Could you check a few things on this model? Use its own coordinates, in mm. Face numbers are marked on the shaded views. A direction names the side the tool comes from. Give positions to 0.01 mm unless a question says otherwise; leave off trailing zeros. Loops run counter-clockwise (first coordinate to the right, second up) from the corner with the lowest first, then second, coordinate; pieces in that order, holes last. Notation, with made-up numbers: (88.25, 43) -> (105.25, 43) arc R16 ccw to (105.25, 50) -> close; hole circle Ø3 at (75, 75.5). An arc over 180 degrees is marked (long way). Put each result on its own line as item: value.
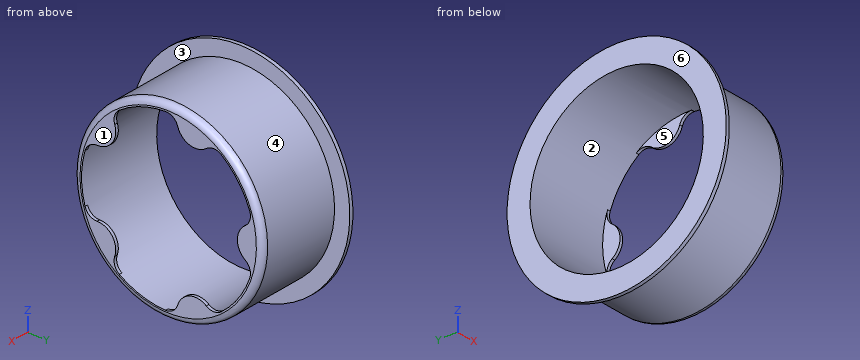
```python
from build123d import *

# Parameters (mm, degrees)
SKETCH_3_R          = 19
CUT_EXTRUDE_1_DEPTH = 0.6
EXTRUDE_1_DEPTH     = 0.5
FILLET_1_R          = 2
FILLET_2_R          = 1


with BuildPart() as part:
    # 草图2 → 旋转1 (revolve)
    with BuildSketch(Plane(origin=(0, 0, 0), x_dir=(1, 0, 0), z_dir=(0, 1, 0)), mode=Mode.PRIVATE) as revolve_1_sk:
        Polygon((-7.6, 14.15), (-7.6, 17.9), (-7, 17.9), (-7, 15.4), (7, 15.4), (7, 17.9), (7.6, 17.9), (7.6, 14.15), align=None)
    revolve(revolve_1_sk.sketch.rotate(Axis((-68.553057404, 0, 0), (1, 0, 0)), 180), axis=Axis((-68.553057404, 0, 0), (1, 0, 0)))

    # 草图3 → 切除-拉伸1 (cut)
    with BuildSketch(Plane(origin=(7.6, 0, 0), x_dir=(0, 0, -1), z_dir=(1, 0, 0))):
        Circle(SKETCH_3_R)
    extrude(amount=-CUT_EXTRUDE_1_DEPTH, mode=Mode.SUBTRACT)

    # 草图4 → 凸台-拉伸1 (add)
    with BuildSketch(Plane(origin=(7, 0, 0), x_dir=(0, 0, -1), z_dir=(1, 0, 0))):
        with BuildLine():
            ThreePointArc((-12.378887951, 7.159129353), (-13.600108183, 4.41894302), (-14.222761377, 1.484270465))
            ThreePointArc((-14.222761377, 1.484270465), (-10.746938634, 3.491892036), (-12.378887951, 7.159129353))
        make_face()
        with BuildLine():
            ThreePointArc((-2.983449874, 13.985314685), (0, 11.3), (2.983449874, 13.985314685))
            ThreePointArc((2.983449874, 13.985314685), (0, 14.3), (-2.983449874, 13.985314685))
        make_face()
        with BuildLine():
            ThreePointArc((12.378887951, 7.159129353), (10.746938634, 3.491892036), (14.222761377, 1.484270465))
            ThreePointArc((14.222761377, 1.484270465), (13.600108183, 4.41894302), (12.378887951, 7.159129353))
        make_face()
        with BuildLine():
            ThreePointArc((10.634023371, -9.560729415), (6.641973351, -9.141892036), (5.80670007, -13.067985089))
            ThreePointArc((5.80670007, -13.067985089), (8.405329108, -11.56894302), (10.634023371, -9.560729415))
        make_face()
        with BuildLine():
            ThreePointArc((-5.80670007, -13.067985089), (-6.641973351, -9.141892036), (-10.634023371, -9.560729415))
            ThreePointArc((-10.634023371, -9.560729415), (-8.405329108, -11.56894302), (-5.80670007, -13.067985089))
        make_face()
    extrude(amount=-EXTRUDE_1_DEPTH)

    # 圆角1
    # the kernel refuses this fillet: 2 mm, written as the material it adds along each edge
    with BuildSketch(Plane(origin=(7, 13.836101399, -2.963916005), x_dir=(0, -0.2740436561087124, -0.9617172529109426), z_dir=(-1, 0, 0)), Plane(origin=(7, 1.456738837, -14.074814811), x_dir=(0, -0.9993316071526622, -0.03655597004153086), z_dir=(-1, 0, 0)), Plane(origin=(7, -12.935787284, -5.734797933), x_dir=(0, -0.3435772431436893, 0.9391244209335534), z_dir=(-1, 0, 0)), Plane(origin=(7, -9.45149505, 10.53051477), x_dir=(0, 0.7869891931288754, 0.6169667818435298), z_dir=(-1, 0, 0)), Plane(origin=(7, 7.094442099, 12.24301398), x_dir=(0, 0.8299633132761892, -0.5578179798246109), z_dir=(-1, 0, 0))) as fillet_1_piece_1:
        with BuildLine():
            CenterArc((1.749454913, 1.995570291), FILLET_1_R, 199.01971257, 74.794373043)
            ThreePointArc((-0.141358103, 1.34378341), (0.005960171, 0.6799537), (0, 0))
            ThreePointArc((0, 0), (0.941246655, -0.031340193), (1.88249331, 0))
        make_face()
    extrude(amount=0.5)
    with BuildSketch(Plane(origin=(7, 13.836101399, 2.963916005), x_dir=(0, -0.2740436561087127, 0.9617172529109423), z_dir=(-1, 0, 0)), Plane(origin=(7, 7.094442099, -12.24301398), x_dir=(0, 0.8299633132761899, 0.5578179798246101), z_dir=(-1, 0, 0)), Plane(origin=(7, -9.45149505, -10.53051477), x_dir=(0, 0.7869891931288755, -0.6169667818435297), z_dir=(-1, 0, 0)), Plane(origin=(7, -12.935787284, 5.734797933), x_dir=(0, -0.34357724314368965, -0.9391244209335534), z_dir=(-1, 0, 0)), Plane(origin=(7, 1.456738837, 14.074814811), x_dir=(0, -0.9993316071526621, 0.03655597004153149), z_dir=(-1, 0, 0))) as fillet_1_piece_2:
        with BuildLine():
            CenterArc((1.749454913, -1.995570291), FILLET_1_R, 86.185914387, 74.794373043)
            ThreePointArc((-0.141358103, -1.34378341), (0.005960171, -0.6799537), (0, 0))
            ThreePointArc((0, 0), (0.941246655, 0.031340193), (1.88249331, 0))
        make_face()
    extrude(amount=0.5)

    # 圆角2
    fillet_2_edges = [part.edges().sort_by_distance(p)[0] for p in [
        (7, 0, -15.4),
    ]]
    fillet(fillet_2_edges, radius=FILLET_2_R)


solid = part.part
```
1. If we section it at B-B (x = 3): List the corners of the cut face in (y, z) for me, then the cut area to 3 significant figures.
Recorded:
outline: circle Ø30.8 at (0, 0); hole circle Ø28.3 at (0, 0)
area: 116 mm^2
2. If we section it at D-D (y = 16.5): List the corners of the cut face in (x, z) for me.
Recorded:
outline: (-7.6, -6.94) -> (-7, -6.94) -> (-7, 6.94) -> (-7.6, 6.94) -> close
3. Thinking about a two-plate mould opening in Z: for the marked faces 4, 5 and 6, which applies, pulls with the +Z half, pulls with the -Z half, needs draft (parallel to the pull), parting line crosses it, or undercut?
Recorded:
face 4: parting line crosses it
face 5: undercut
face 6: needs draft
4. If we section it at A-A (z = 0): List the corners of the cut face in (x, y) for me.
Recorded:
outline: (-7.6, -17.9) -> (-7, -17.9) -> (-7, -15.4) -> (6, -15.4) arc R1 ccw to (7, -14.4) -> (7, -14.15) -> (-7.6, -14.15) -> close; (-7.6, 14.15) -> (6.5, 14.15) -> (6.5, 11.3) -> (7, 11.3) -> (7, 14.4) arc R1 ccw to (6, 15.4) -> (-7, 15.4) -> (-7, 17.9) -> (-7.6, 17.9) -> close
5. I need wall thicknesses on line 1 (Y direction, x = 3, z = 0); line 2 (Z direction, x = 6.25, y = -10); line 3 (X direction, y = -10.5, z = -7). Which ranges of each line are inside material? Lowest first, please.
Recorded:
line 1: y = -15.4 to -14.15, 14.15 to 15.4
line 2: z = -11.67 to -10.01, 10.01 to 11.67
line 3: x = 6.5 to 7
6. I'm going to push flat-ended pins straight in: pin 1 (3 mm diameter, centred on y = 9.5, z = 4, fed in from -X); pin 2 (6 mm diameter, centred on x = 4.5, y = -13.5, fed in from +Z); pin 3 (5 mm diameter, centred on x = -1.5, z = 0, fed in from +Y); pin 4 (1.7 mm diameter, centred on y = -9.5, z = 7, fed in from -X). Where does each tip first touch, or does it pass through?
Recorded:
pin 1: passes through
pin 2: stops at z = 11.27
pin 3: stops at y = 15.4
pin 4: stops at x = 6.5
7. For the marked faces 1, 2 and 3, which set-ups out of +Z, -Z, +X, -X, +Y, -Y let a thin tool reach every point of the face, with its end or its side?
Recorded:
face 1: +Z, -Z, +X, +Y, -Y
face 2: -X
face 3: +X
